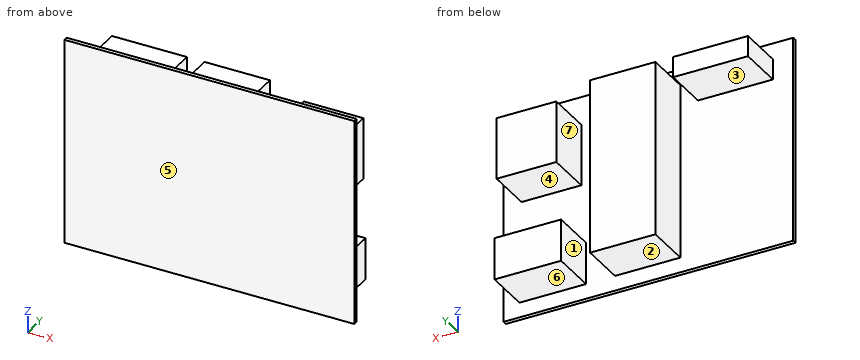
from build123d import *

# Parameters (mm, degrees)
SKETCH1_W           = 70
SKETCH1_H           = 50
BOSS_EXTRUDE1_DEPTH = 1
SKETCH2_W           = 15.79200929
SKETCH2_H           = 42.472572931
SKETCH2_W_2         = 16.080447816
SKETCH2_H_2         = 10.167458036
SKETCH2_W_3         = 14.421926292
SKETCH2_H_3         = 14.926693712
SKETCH2_W_4         = 18.099517497
SKETCH2_H_4         = 4.975564571
BOSS_EXTRUDE2_DEPTH = 12


with BuildPart() as part:
    # Sketch1 → Boss-Extrude1 (new body)
    with BuildSketch(Plane(origin=(0, 0, 0), x_dir=(1, 0, 0), z_dir=(0, 1, 0))):
        with Locations((3.189448441, 12.661870504)):
            Rectangle(SKETCH1_W, SKETCH1_H)
    extrude(amount=BOSS_EXTRUDE1_DEPTH)

    # Sketch2 → Boss-Extrude2 (add)
    with BuildSketch(Plane(origin=(0, 0, 0), x_dir=(1, 0, 0), z_dir=(0, 1, 0))):
        with Locations((3.333667704, 12.806089767)):
            Rectangle(SKETCH2_W, SKETCH2_H)
        with Locations((26.264530509, 28.958647214)):
            Rectangle(SKETCH2_W_2, SKETCH2_H_2)
        with Locations((26.58902385, 1.917535416)):
            Rectangle(SKETCH2_W_3, SKETCH2_H_3)
        with Locations((-17.866563946, -5.942414413)):
            Rectangle(SKETCH2_W_4, SKETCH2_H_4)
    extrude(amount=BOSS_EXTRUDE2_DEPTH)


solid = part.part
Can you work these out from the model? Positions are in its coordinate system, mm. Face numbers are marked on the shaded views. A direction names the side the tool comes from. Coordinates: 2 decimals unless noted, no trailing zeros. Loops run counter-clockwise (first coordinate to the right, second up) from the corner with the lowest first, then second, coordinate; pieces in that order, holes last. Notation, with made-up numbers: (8.5, 72.5) - (22.5, 72.5) arc R22 cw to (22.5, 97.5) - close; hole circle Ø8 at (80.5, -29). An arc over 180 degrees is marked (long way). Put each result on its own line as item: value. Start each with the question number.
Item 1: If we mould it in two halves opening along X, with no side actions, what happens to the marked faces 1 and 2? For each: +X half, -X half, draft (parallel to the pull), parting line (faces both ways), or undercut.
Item 2: Suppose I cut it at D-D (z = -13). Please give me the cut outline in (x, y), and give its area (3 significant figures).
Item 3: Suppose I cut it at C-C (x = -14). Please give me the cut outline in (y, z).
Item 4: Suppose I cut it at A-A (y = 5.25). Please give me the cut outline in (x, z), and give its area (3 significant figures).
Item 5: Which directions (+Z, -Z, +X, -X, +Y, -Y) give clear straight access to the entire face, cutting with the end or side of a thin tool? Please do the marked faces 3, 4, 5, 6 and 7.
Item 6: For pin 1 (5 mm diameter, centred on y = 9.5, z = -25.5, fed in from -X); pin 2 (5.5 mm diameter, centred on y = 9, z = 4.5, fed in from +X); pin 3 (5.5 mm diameter, centred on x = 27.5, y = 8, fed in from +Z), each with a flat end and sliding along its axis, tell me the tip position at first contact or that it passes through.
Item 7: Suppose I cut it at B-B (z = -31). Please give me the cut outline in (x, y), and give its area (3 significant figures).
Item 8: If I drill on line 1 along X through (y, z) = (2.5, 8); line 2 along X through (y, z) = (8.5, -6); line 3 along Z through (x, y) = (30, 3.5), over which ranges is the centre line in solid material (lowest first)?
Here are the results:
1. face 1: undercut
1. face 2: draft
2. outline: (-31.81, 0) - (38.19, 0) - (38.19, 1) - (11.23, 1) - (11.23, 12) - (-4.56, 12) - (-4.56, 1) - (-31.81, 1) - close
2. area: 244 mm²
3. outline: (0, -37.66) - (1, -37.66) - (1, 3.45) - (12, 3.45) - (12, 8.43) - (1, 8.43) - (1, 12.34) - (0, 12.34) - close
4. outline: (-26.92, 3.45) - (-8.82, 3.45) - (-8.82, 8.43) - (-26.92, 8.43) - close; (-4.56, -34.04) - (11.23, -34.04) - (11.23, 8.43) - (-4.56, 8.43) - close; (18.22, -34.04) - (34.3, -34.04) - (34.3, -23.87) - (18.22, -23.87) - close; (19.38, -9.38) - (33.8, -9.38) - (33.8, 5.55) - (19.38, 5.55) - close
4. area: 1,140 mm²
5. face 3: -Z, -X, +Y
5. face 4: +X, +Y
5. face 5: +Z, -Z, +X, -X, -Y
5. face 6: -Z, +X, -X, +Y
5. face 7: +Z, +Y
6. pin 1: x = -4.56
6. pin 2: x = 33.8
6. pin 3: z = 5.55
7. outline: (-31.81, 0) - (38.19, 0) - (38.19, 1) - (34.3, 1) - (34.3, 12) - (18.22, 12) - (18.22, 1) - (11.23, 1) - (11.23, 12) - (-4.56, 12) - (-4.56, 1) - (-31.81, 1) - close
7. area: 421 mm²
8. line 1: -26.92 to -8.82, -4.56 to 11.23
8. line 2: -4.56 to 11.23, 19.38 to 33.8
8. line 3: -34.04 to -23.87, -9.38 to 5.55
